```python
from build123d import *

# Parameters (mm, degrees)
EXTRUDE_THIN1_DEPTH = 53
SKETCH2_R           = 10
BOSS_EXTRUDE1_DEPTH = 5
SKETCH4_R           = 7.5
BOSS_EXTRUDE2_DEPTH = 33
SKETCH5_W           = 43
SKETCH5_H           = 25
BOSS_EXTRUDE3_DEPTH = 5
SKETCH6_R           = 1.5
CUT_EXTRUDE1_DEPTH  = 5


with BuildPart() as part:
    # Sketch1 → Extrude-Thin1 (new body)
    with BuildSketch(Plane.XY):
        Polygon((0, 25), (0, 0), (25, 0), (25, 2), (2, 2), (2, 25), align=None)
    extrude(amount=EXTRUDE_THIN1_DEPTH)

    # Sketch2 → Boss-Extrude1 (add)
    with BuildSketch(Plane.ZY):
        with Locations((15, 12.5)):
            Circle(SKETCH2_R)
        with Locations((38, 12.5)):
            Circle(SKETCH2_R)
    extrude(amount=BOSS_EXTRUDE1_DEPTH)

    # Sketch4 → Boss-Extrude2 (add)
    with BuildSketch(Plane.ZY.offset(5)):
        with Locations((38, 12.5)):
            Circle(SKETCH4_R)
        with Locations((15, 12.5)):
            Circle(SKETCH4_R)
    extrude(amount=-BOSS_EXTRUDE2_DEPTH)

    # Sketch5 → Boss-Extrude3 (add)
    with BuildSketch(Plane(origin=(28, 0, 0), x_dir=(0, 0, -1), z_dir=(1, 0, 0))):
        with Locations((-26.5, 17.5)):
            Rectangle(SKETCH5_W, SKETCH5_H)
    extrude(amount=BOSS_EXTRUDE3_DEPTH)

    # Sketch6 → Cut-Extrude1 (cut)
    with BuildSketch(Plane.XZ):
        with Locations(Location((15, 26.5, 0), (0, 0, 270))):
            Circle(SKETCH6_R)
    extrude(amount=-CUT_EXTRUDE1_DEPTH, mode=Mode.SUBTRACT)


solid = part.part
```
Build history of the part. All positions in model axes, mm. A direction names the side the tool comes from. Round coordinates to 2 decimals unless told otherwise and drop trailing zeros. Order: outer loops, then holes, each group sorted by start corner. A loop starts at its lowest first (then second) coordinate and runs counter-clockwise, first axis right, second up. Notation, with made-up numbers: (-33.75, -18.5) -> (-6.75, -18.5) arc R17 ccw to (-6.75, -12.5) -> close; hole circle Ø4 at (-3, 7). An arc over 180 degrees is marked (long way). Answer in a Markdown table with one row per item.
1) Mould opens along X. For faces 1 (the flat face through (28, 20, 27)), 2 (the flat face through (-5, 13, 38)), 3 (the cylindrical face through (-2.46, 2.74, 35.83)), 4 (the cylindrical face through (15, 1, 28)) say: released by +X, released by -X, zero draft, split by the parting line, or undercut.
Values:
| item | result |
|---|---|
| face 1 | undercut |
| face 2 | released by -X |
| face 3 | zero draft |
| face 4 | undercut |
2) Which spindle directions (+Z, -Z, +X, -X, +Y, -Y) get a long thin tool onto all of the face, cutting with end or side? Do faces 5 (the flat face through (30, 17, 5)), 6 (the flat face through (30, 5, 27)), 7 (the flat face through (2, 13, 26)), 8 (the flat face through (1, 25, 26)). Say none if no direction does.
Values:
| item | result |
|---|---|
| face 5 | -Z, +X, +Y, -Y |
| face 6 | +Z, -Z, +X, -Y |
| face 7 | none |
| face 8 | +Z, -Z, -X, +Y |
3) Band-saw the part on A-A on x = 15. Give the cut face in (y, z), and give its area (3 significant figures).
Values:
| item | result |
|---|---|
| outline | (0, 0) -> (2, 0) -> (2, 25) -> (0, 25) -> close; (0, 28) -> (2, 28) -> (2, 53) -> (0, 53) -> close; circle Ø15 at (12.5, 15); circle Ø15 at (12.5, 38) |
| area | 453 mm2 |
4) Band-saw the part on B-B on z = 26.5. Give the cut face in (x, y).
Values:
| item | result |
|---|---|
| outline | (0, 0) -> (13.5, 0) -> (13.5, 2) -> (2, 2) -> (2, 25) -> (0, 25) -> close; (16.5, 0) -> (25, 0) -> (25, 2) -> (16.5, 2) -> close; (28, 5) -> (33, 5) -> (33, 30) -> (28, 30) -> close |
5) Wall check: L1, parallel to X at y = 11.75, z = 7.5; L2, parallel to X at y = 21.75, z = 20.5; L3, parallel to Y at x = 21.5, z = 4. Give the ranges that are in metal, low to high.
Values:
| item | result |
|---|---|
| L1 | -5 to 2, 28 to 33 |
| L2 | 0 to 2, 28 to 33 |
| L3 | 0 to 2 |
6) Band-saw the part on C-C on y = 12.5. Give the cut face in (x, z).
Values:
| item | result |
|---|---|
| outline | (-5, 5) -> (0, 5) -> (0, 0) -> (2, 0) -> (2, 7.5) -> (28, 7.5) -> (28, 5) -> (33, 5) -> (33, 48) -> (28, 48) -> (28, 45.5) -> (2, 45.5) -> (2, 53) -> (0, 53) -> (0, 48) -> (-5, 48) -> (-5, 28) -> (0, 28) -> (0, 25) -> (-5, 25) -> close; hole (2, 22.5) -> (28, 22.5) -> (28, 30.5) -> (2, 30.5) -> close |
7) Pin check, flat tips, straight feed: P1, Ø5.5, axis at x = 31, y = 17.5, coming from the -Z side; P2, Ø11.5, axis at x = 13, z = 18, coming from the +Y side; P3, Ø2, axis at x = 1, z = 38, coming from the +Y side. Stop position of each tip, or through.
Values:
| item | result |
|---|---|
| P1 | z = 5 |
| P2 | y = 20 |
| P3 | y = 25 |
8) Band-saw the part on D-D on x = 7.5. Give the cut face in (y, z), and give its area (3 significant figures).
Values:
| item | result |
|---|---|
| outline | (0, 0) -> (2, 0) -> (2, 53) -> (0, 53) -> close; circle Ø15 at (12.5, 15); circle Ø15 at (12.5, 38) |
| area | 459 mm2 |
